The listing builds one solid part. Answer for the finished solid, in the listing's coordinates (mm). A direction names the side the tool comes from. Coordinates: 2 decimals unless noted, no trailing zeros. Answer in a Markdown table with one row per item.
```python
from build123d import *

# Parameters (mm, degrees)
SKETCH1_W           = 18
SKETCH1_H           = 18
BOSS_EXTRUDE1_DEPTH = 13
FILLET1_R           = 4
SKETCH2_R           = 1.25
CUT_EXTRUDE1_DEPTH  = 18
SKETCH3_R           = 6
CUT_EXTRUDE2_DEPTH  = 10
SKETCH4_R           = 5.25
CUT_EXTRUDE3_DEPTH  = 10
BOSS_EXTRUDE2_START = 6
SKETCH5_R           = 1.75
SKETCH5_R_2         = 1.25
BOSS_EXTRUDE2_DEPTH = 6
FILLET2_R           = 2
CUT_EXTRUDE4_DEPTH  = 2
SKETCH10_W          = 22.06427133
SKETCH10_H          = 21.544432477
CUT_EXTRUDE5_DEPTH  = 1
CHAMFER1_SIZE       = 0.5
CHAMFER2_SIZE       = 0.5
CHAMFER3_SIZE       = 0.5


# Some blends are built 0.0001 mm under size
with BuildPart() as part:
    # Sketch1 → Boss-Extrude1 (new body)
    with BuildSketch(Plane.XY):
        with Locations((-9, 9)):
            Rectangle(SKETCH1_W, SKETCH1_H)
    extrude(amount=BOSS_EXTRUDE1_DEPTH)

    # Fillet1
    fillet1_edges = [part.edges().sort_by_distance(p)[0] for p in [
        (0, 0, 6.5),
        (-18, 0, 6.5),
        (-18, 18, 6.5),
        (0, 18, 6.5),
    ]]
    fillet(fillet1_edges, radius=FILLET1_R)

    # Sketch2 → Cut-Extrude1 (cut)
    with BuildSketch(Plane(origin=(0, 0, 0), x_dir=(-1, 0, 0), z_dir=(0, 0, -1))):
        with Locations((9, 9)):
            Circle(SKETCH2_R)
    extrude(amount=-CUT_EXTRUDE1_DEPTH, mode=Mode.SUBTRACT)

    # Sketch3 → Cut-Extrude2 (cut)
    with BuildSketch(Plane(origin=(0, 0, 0), x_dir=(-1, 0, 0), z_dir=(0, 0, -1))):
        with BuildLine():
            Line((1, 14), (1, 4))
            ThreePointArc((1, 4), (1.878679656, 1.878679656), (4, 1))
            Line((4, 1), (14, 1))
            ThreePointArc((14, 1), (16.121320344, 1.878679656), (17, 4))
            Line((17, 4), (17, 14))
            ThreePointArc((17, 14), (16.121320344, 16.121320344), (14, 17))
            Line((14, 17), (4, 17))
            ThreePointArc((4, 17), (1.878679656, 16.121320344), (1, 14))
        make_face()
        with Locations((9, 9)):
            Circle(SKETCH3_R, mode=Mode.SUBTRACT)
    extrude(amount=-CUT_EXTRUDE2_DEPTH, mode=Mode.SUBTRACT)

    # Sketch4 → Cut-Extrude3 (cut)
    with BuildSketch(Plane(origin=(0, 0, 0), x_dir=(-1, 0, 0), z_dir=(0, 0, -1))):
        with Locations((9, 9)):
            Circle(SKETCH4_R)
    extrude(amount=-CUT_EXTRUDE3_DEPTH, mode=Mode.SUBTRACT)

    # Sketch5 → Boss-Extrude2 (add)
    with BuildSketch(Plane(origin=(0, 0, 10), x_dir=(-1, 0, 0), z_dir=(0, 0, -1)).offset(BOSS_EXTRUDE2_START)):
        with Locations((9, 9)):
            Circle(SKETCH5_R)
        with Locations((9, 9)):
            Circle(SKETCH5_R_2, mode=Mode.SUBTRACT)
    extrude(amount=-BOSS_EXTRUDE2_DEPTH)

    # Sketch7 → Cut-Revolve4 (revolve, cut)
    with BuildSketch(Plane(origin=(0, 9, 0), x_dir=(1, 0, 0), z_dir=(0, 1, 0))):
        with BuildLine():
            Line((-9, -10.9), (-9, -43.1))
            ThreePointArc((-9, -43.1), (7.1, -27), (-9, -10.9))
        make_face()
    revolve(axis=Axis((-9, 9, 0), (0, 0, 1)), mode=Mode.SUBTRACT)

    # Fillet2
    # the kernel refuses this fillet: 2 mm, written as the material it takes off along each edge
    with BuildSketch(Plane(origin=(0, 14, 13), x_dir=(-1, 0, 0), z_dir=(0, -1, 0)), Plane(origin=(-14, 18, 13), x_dir=(0, -1, 0), z_dir=(1, 0, 0)), Plane(origin=(-18, 4, 13), x_dir=(1, 0, 0), z_dir=(0, 1, 0))) as fillet2_piece_1:
        with BuildLine():
            CenterArc((FILLET2_R, FILLET2_R), FILLET2_R, 180, 90)
            Line((0, FILLET2_R), (0, 0))
            Line((0, 0), (FILLET2_R, 0))
        make_face()
    extrude(amount=10, mode=Mode.SUBTRACT)
    with BuildSketch(Plane(origin=(-4, 0, 13), x_dir=(0, 0, -1), z_dir=(-1, 0, 0))) as fillet2_piece_2:
        with BuildLine():
            CenterArc((FILLET2_R, -FILLET2_R), FILLET2_R, 90, 90)
            Line((0, -FILLET2_R), (0, 0))
            Line((0, 0), (FILLET2_R, 0))
        make_face()
    extrude(amount=10, mode=Mode.SUBTRACT)
    with BuildSketch(Plane(origin=(-4, 14, 13), x_dir=(0, 1, 0), z_dir=(-1, 0, 0))) as fillet2_piece_3:
        with BuildLine():
            CenterArc((4 - FILLET2_R, FILLET2_R), FILLET2_R, 270, 90)
            Line((4, FILLET2_R), (4, 0))
            Line((4, 0), (4 - FILLET2_R, 0))
        make_face()
    revolve(axis=Axis((-4, 14, 13), (0, 0, -1)), revolution_arc=90, mode=Mode.SUBTRACT)
    with BuildSketch(Plane(origin=(-14, 14, 13), x_dir=(-1, 0, 0), z_dir=(0, -1, 0))) as fillet2_piece_4:
        with BuildLine():
            CenterArc((4 - FILLET2_R, FILLET2_R), FILLET2_R, 270, 90)
            Line((4, FILLET2_R), (4, 0))
            Line((4, 0), (4 - FILLET2_R, 0))
        make_face()
    revolve(axis=Axis((-14, 14, 13), (0, 0, -1)), revolution_arc=90, mode=Mode.SUBTRACT)
    with BuildSketch(Plane(origin=(-14, 4, 13), x_dir=(0, -1, 0), z_dir=(1, 0, 0))) as fillet2_piece_5:
        with BuildLine():
            CenterArc((4 - FILLET2_R, FILLET2_R), FILLET2_R, 270, 90)
            Line((4 - FILLET2_R, 0), (4, 0))
            Line((4, 0), (4, FILLET2_R))
        make_face()
    revolve(axis=Axis((-14, 4, 13), (0, 0, -1)), revolution_arc=90, mode=Mode.SUBTRACT)
    with BuildSketch(Plane(origin=(-4, 4, 13), x_dir=(0, -1, 0), z_dir=(-1, 0, 0))) as fillet2_piece_6:
        with BuildLine():
            CenterArc((4 - FILLET2_R, -FILLET2_R), FILLET2_R, 0, 90)
            Line((4 - FILLET2_R, 0), (4, 0))
            Line((4, 0), (4, -FILLET2_R))
        make_face()
    revolve(axis=Axis((-4, 4, 13), (0, 0, 1)), revolution_arc=90, mode=Mode.SUBTRACT)
    with BuildSketch(Plane(origin=(-9, 9, 13), x_dir=(1, 0, 0), z_dir=(0, 1, 0))) as fillet2_piece_7:
        with BuildLine():
            CenterArc((8.462269199, 2), FILLET2_R, 242.126002653, 27.873997347)
            ThreePointArc((7.527211829, 0.232044199), (7.73971142, 0.117608407), (7.950471684, 0))
            Line((7.950471684, 0), (8.462269199, 0))
        make_face()
    revolve(axis=Axis((-9, 9, 13), (0, 0, -1)), mode=Mode.SUBTRACT)

    # Sketch9 → Cut-Extrude4 (cut)
    with BuildSketch(Plane(origin=(0, 0, 0), x_dir=(-1, 0, 0), z_dir=(0, 0, -1))):
        with BuildLine():
            Line((16.707106781, 15.292893219), (17.445719569, 16.031506006))
            ThreePointArc((17.445719569, 16.031506006), (16.828427125, 16.828427125), (16.031506006, 17.445719569))
            Line((16.031506006, 17.445719569), (15.292893219, 16.707106781))
            ThreePointArc((15.292893219, 16.707106781), (16.121320344, 16.121320344), (16.707106781, 15.292893219))
        make_face()
    extrude(amount=-CUT_EXTRUDE4_DEPTH, mode=Mode.SUBTRACT)

    # Sketch10 → Cut-Extrude5 (cut)
    with BuildSketch(Plane(origin=(0, 0, 0), x_dir=(-1, 0, 0), z_dir=(0, 0, -1))):
        with Locations((9.251838168, 8.653440765)):
            Rectangle(SKETCH10_W, SKETCH10_H)
    extrude(amount=-CUT_EXTRUDE5_DEPTH, mode=Mode.SUBTRACT)

    # Chamfer1
    chamfer1_edges = [part.edges().sort_by_distance(p)[0] for p in [
        (-1, 9, 1),
        (-1.878679656, 16.121320344, 1),
        (-9, 17, 1),
        (-14.662827148, 16.925860587, 1),
        (-16.925860587, 14.662827148, 1),
        (-17, 9, 1),
        (-16.121320344, 1.878679656, 1),
        (-9, 1, 1),
        (-1.878679656, 1.878679656, 1),
        (-3, 9, 1),
    ]]
    chamfer(chamfer1_edges, length=CHAMFER1_SIZE)

    # Chamfer2
    chamfer2_edges = [part.edges().sort_by_distance(p)[0] for p in [
        (-7.75, 9, 4),
    ]]
    chamfer(chamfer2_edges, length=CHAMFER2_SIZE - 0.0001)  # a hair under: the kernel refuses the full size

    # Chamfer3
    # the kernel refuses this chamfer: 0.543867406, 0.5 mm, written as the material it takes off along each edge
    with BuildSketch(Plane(origin=(-9, 9, 10.948598192), x_dir=(-1, 0, 0), z_dir=(0, -1, 0))) as chamfer3_piece_1:
        with BuildLine():
            Line((1.25, CHAMFER3_SIZE), (1.802636138, -0.052636138))
            ThreePointArc((1.802636138, -0.052636138), (1.534897868, -0.024733766), (1.25, 0))
            Line((1.25, 0), (1.25, CHAMFER3_SIZE))
        make_face()
    revolve(axis=Axis((-9, 9, 10.948598192), (0, 0, -1)), revolution_arc=180, mode=Mode.SUBTRACT)
    with BuildSketch(Plane(origin=(-9, 9, 10.948598192), x_dir=(1, 0, 0), z_dir=(0, 1, 0))) as chamfer3_piece_2:
        with BuildLine():
            Line((1.25, CHAMFER3_SIZE), (1.802636138, -0.052636138))
            ThreePointArc((1.802636138, -0.052636138), (1.534897868, -0.024733766), (1.25, 0))
            Line((1.25, 0), (1.25, CHAMFER3_SIZE))
        make_face()
    revolve(axis=Axis((-9, 9, 10.948598192), (0, 0, -1)), revolution_arc=180, mode=Mode.SUBTRACT)


solid = part.part
```
(1) Find the intervals of material crossed by line 1 along Y through (x, z) = (-9, 3.5); line 2 along Y through (x, z) = (-9, 8.7); line 3 along X through (y, z) = (11.75, 6), in increasing order. Write a range as from..to.
Check values:
| item | result |
|---|---|
| line 1 | 0..1, 3..3.75, 14.25..15, 17..18 |
| line 2 | 0..1, 3..3.75, 7.25..7.75, 10.25..10.75, 14.25..15, 17..18 |
| line 3 | -18..-17, -14.33..-13.47, -4.53..-3.67, -1..0 |
(2) Which of the six approach directions +Z, -Z, +X, -X, +Y, -Y give full straight-line access (tool end or side, diameter ignored) to faces 1 (the cylindrical face through (-8.079, 9.845, 7.433)), 2 (the conical face through (-1.754, 16.197, 1.358))?
Check values:
| item | result |
|---|---|
| face 1 | +Z, -Z |
| face 2 | -Z |
(3) Flat-ended cylindrical pins translate along their axes: pin 1 (1.1 mm diameter, centred on x = -16.5, y = 16, fed in from -Z); pin 2 (3 mm diameter, centred on x = -9, y = 9, fed in from -Z); pin 3 (9.5 mm diameter, centred on x = -9, y = 9, fed in from +Z). Find the tip coordinate at first contact, or state that the pin passes through.
Check values:
| item | result |
|---|---|
| pin 1 | z = 2 |
| pin 2 | z = 4.25 |
| pin 3 | z = 11.62 |
(4) For a pull along X with two mould halves and no side action, classify faces 3 (the flat face through (-9, 17, 6)), 4 (the flat face through (-15.1, 2.9, 13)), 5 (the cylindrical face through (-17.65, 8.93, 12.13)), 6 (the cylindrical face through (-1.86, 1.9, 5.69)) as released by +X, released by -X, zero draft, split by the parting line, or undercut.
Check values:
| item | result |
|---|---|
| face 3 | undercut |
| face 4 | zero draft |
| face 5 | released by -X |
| face 6 | undercut |
